Solid Edge part; units mm, degrees
sketch "Sketch1" plane through (0, 0, 0) normal (0, 0, 1) x (1, 0, 0)
  line L0 (0, 0) -> (0, 19.812)
  line L1 (0, 19.812) -> (39.624, 19.812)
  line L2 (39.624, 19.812) -> (39.624, 0)
  line L3 (39.624, 0) -> (0, 0)
  dimension "D1" = 39.624
extrude "Protrusion1" add sketch "Sketch1" along normal blind 36.576
sketch "Sketch2" plane through (19.812, 9.906, 26.416) normal (0, 0, 1) x (1, 0, 0)
  line L0 (-26.2372, -9.906) -> (-26.2372, 9.906)
  line L1 (-26.2372, 9.906) -> (26.5948, 9.906)
  line L2 (26.5948, 9.906) -> (26.5948, -9.906)
  line L3 (26.5948, -9.906) -> (-26.2372, -9.906)
extrude "ExtrudedProtrusion_2" add sketch "Sketch2" along normal blind 2.54
sketch "Sketch3" plane through (19.812, 9.906, 36.576) normal (0, 0, 1) x (1, 0, 0)
  circle A0 centre (-10.033, 0) radius 2.54
extrude "ExtrudedProtrusion_3" add sketch "Sketch3" along normal blind 3.048
hole "Hole_1" at (-3.6312, 4.826, 28.956) direction (0, 0, -1) diameter 4.572 end through all
hole "Hole1" at (43.6128, 4.826, 28.956) direction (0, 0, -1) diameter 4.572 end through all
hole "Hole2" at (43.6128, 14.986, 28.956) direction (0, 0, -1) diameter 4.572 end through all
hole "Hole3" at (-3.6312, 14.986, 28.956) direction (0, 0, -1) diameter 4.572 end through all
properties part number "HARDWARE"
The listing builds one solid part. Answer for the finished solid, in the listing's coordinates (mm). A direction names the side the tool comes from. Coordinates: 2 decimals unless noted, no trailing zeros. Order: outer loops, then holes, each group sorted by start corner. A loop starts at its lowest first (then second) coordinate and runs counter-clockwise, first axis right, second up. Notation, with made-up numbers: M 29,58 L 87,58 A16 cw 87,86 Z; hole C 12,-25.5 d10. An arc over 180 degrees is marked long. Use CSV: the item, a comma, the result in double quotes.
Q1. Section D-D (y = 11.5) is taken. Determine the outline of the cut face in (x, z), then the cut area to 3 significant figures.
Here are the results:
outline,"M -6.43,26.42 L 0,26.42 L 0,0 L 39.62,0 L 39.62,26.42 L 46.41,26.42 L 46.41,28.96 L 39.62,28.96 L 39.62,36.58 L 11.76,36.58 L 11.76,39.62 L 7.8,39.62 L 7.8,36.58 L 0,36.58 L 0,28.96 L -6.43,28.96 Z"
area,"1,490 mm2"
Q2. Section A-A (y = 3.5) is taken. Determine the outline of the cut face in (x, z), then the cut area to 3 significant figures.
Here are the results:
outline,"M -6.43,26.42 L -5.49,26.42 L -5.49,28.96 L -6.43,28.96 Z; M -1.77,26.42 L 0,26.42 L 0,0 L 39.62,0 L 39.62,26.42 L 41.75,26.42 L 41.75,28.96 L 39.62,28.96 L 39.62,36.58 L 0,36.58 L 0,28.96 L -1.77,28.96 Z; M 45.47,26.42 L 46.41,26.42 L 46.41,28.96 L 45.47,28.96 Z"
area,"1,460 mm2"
Q3. Straight lines are drawn through the part: L1, parallel to X at y = 16.5, z = 28; L2, parallel to X at y = 5.5, z = 4; L3, parallel to Z at x = 26, y = 18. For each, find the intervals that lie inside material, in ascending order.
Here are the results:
L1,"-6.43 to -5.34, -1.92 to 41.9, 45.33 to 46.41"
L2,"0 to 39.62"
L3,"0 to 36.58"
Q4. Determine the mould class of faces 5 (the cylindrical face through (9.448, 7.388, 38.079)), 6 (the cylindrical face through (45.88, 5.12, 27.7)), 7 (the flat face through (0, 10, 33)), 8 (the cylindrical face through (45.88, 15.28, 27.7)) for opening direction X: pulls with the +X half, pulls with the -X half, needs draft (parallel to the pull), parting line crosses it, or undercut.
Here are the results:
face 5,"parting line crosses it"
face 6,"undercut"
face 7,"pulls with the -X half"
face 8,"undercut"
Q5. A tool of negligible diameter and unlimited length cuts with its end or side. For faces 1 (the flat face through (0, 10, 13)), 2 (the flat face through (43, 10, 26.416)), 3 (the flat face through (39.624, 10, 33)), 4 (the flat face through (-3, 10, 28.956)), from which of +Z, -Z, +X, -X, +Y, -Y can it reach the whole face along a straight path? Write none if from no direction.
Here are the results:
face 1,"-Z, -X, +Y, -Y"
face 2,"-Z, +X, +Y, -Y"
face 3,"+Z, +X, +Y, -Y"
face 4,"+Z, -X, +Y, -Y"
Q6. Section C-C (z = 7) is taken. Determine the outline of the cut face in (x, y), then the cut area to 3 significant figures.
Here are the results:
outline,"M 0,0 L 39.62,0 L 39.62,19.81 L 0,19.81 Z"
area,"785 mm2"
Q7. Given pin 1 Ø1 at (y, z) = (5, 20.5) entering from -X; pin 2 Ø6 at (x, y) = (43.61, 4.83) entering from +Z; pin 3 Ø3 at (x, z) = (29.5, 26.5) entering from -Y; pin 4 Ø6 at (x, y) = (27, 10) entering from +Z, each flat-ended and moving along its own axis, determine where each tip first touches the part or whether it passes through.
Here are the results:
pin 1,"x = 0"
pin 2,"z = 28.96"
pin 3,"y = 0"
pin 4,"z = 36.58"
Q8. Section B-B (z = 27) is taken. Determine the outline of the cut face in (x, y), then the cut area to 3 significant figures.
Here are the results:
outline,"M -6.43,0 L 46.41,0 L 46.41,19.81 L -6.43,19.81 Z; hole C -3.63,4.83 d4.57; hole C -3.63,14.99 d4.57; hole C 43.61,4.83 d4.57; hole C 43.61,14.99 d4.57"
area,"981 mm2"
